Could you check a few things on this drawing? It's one solid part, dimensions in mm from its lowest x, y, z. Round coordinates to 2 decimals unless told otherwise and drop trailing zeros. Write each loop counter-clockwise with the first axis right and the second up, starting at its lowest first coordinate (ties: lowest second). Pieces come first, ordered by that corner, then holes. Notation, with made-up numbers: (-19.75, 2) - (36.25, 2) arc R11 ccw to (36.25, 10) - close; hole circle Ø3 at (63.25, -30). An arc over 180 degrees is marked (long way). Use one line per item in the form item = value. Start each with the question number.
1. I want a section at A-A, the plane z = 5. List the corners of the cut face in (x, y) for me, plus the area to 3 significant figures.
2. I want a section at B-B, the plane x = 36. List the corners of the cut face in (y, z) for me.
3. I want a section at C-C, the plane y = 0.85. List the corners of the cut face in (x, z) for me, plus the area to 3 significant figures.
4. If I drill on line 1 along Z through (x, y) = (36, 0.4); line 2 along X through (y, z) = (0.45, 5); line 3 along Z through (x, y) = (7, 0.85), over which ranges is the centre line in solid material (lowest first)?
5. I want a section at D-D, the plane x = 16.5. List the corners of the cut face in (y, z) for me, plus the area to 3 significant figures.
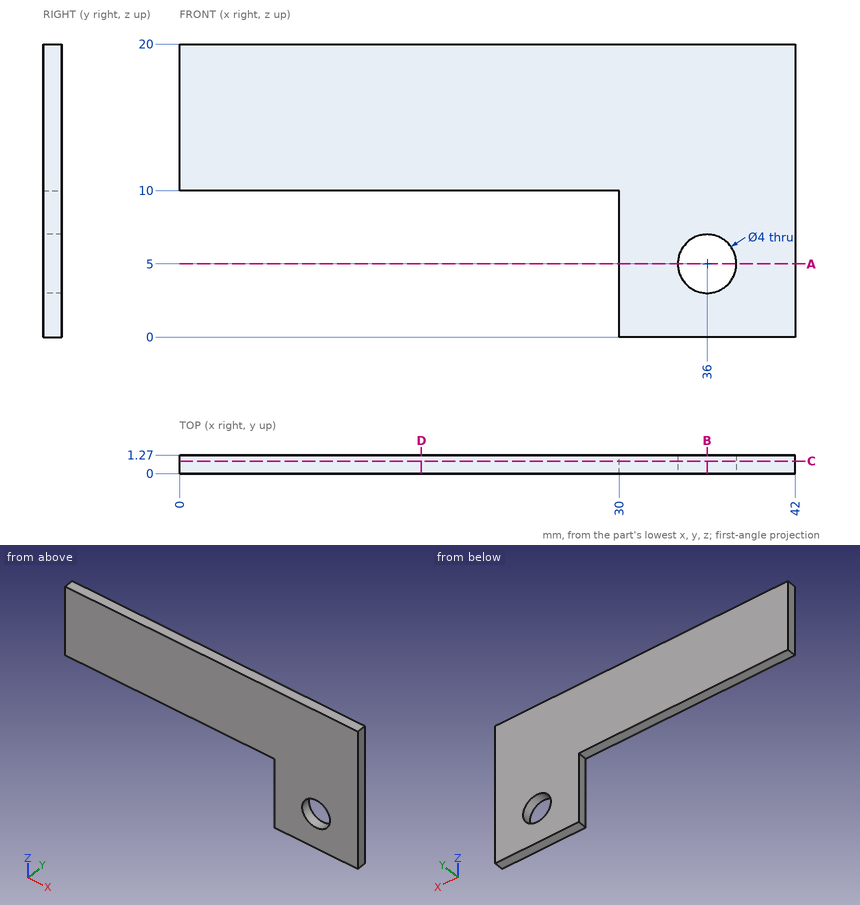
Model answer:
q1.outline = (30, 0) - (34, 0) - (34, 1.27) - (30, 1.27) - close; (38, 0) - (42, 0) - (42, 1.27) - (38, 1.27) - close
q1.area = 10.2 mm2
q2.outline = (0, 0) - (1.27, 0) - (1.27, 3) - (0, 3) - close; (0, 7) - (1.27, 7) - (1.27, 20) - (0, 20) - close
q3.outline = (0, 10) - (30, 10) - (30, 0) - (42, 0) - (42, 20) - (0, 20) - close; hole circle Ø4 at (36, 5)
q3.area = 527 mm2
q4.line_1 = 0 to 3, 7 to 20
q4.line_2 = 30 to 34, 38 to 42
q4.line_3 = 10 to 20
q5.outline = (0, 10) - (1.27, 10) - (1.27, 20) - (0, 20) - close
q5.area = 12.7 mm2
